Verification items for the finished model (mm, model axes). A direction names the side the tool comes from. Coordinates: 2 decimals unless noted, no trailing zeros. Order: outer loops, then holes, each group sorted by start corner. A loop starts at its lowest first (then second) coordinate and runs counter-clockwise, first axis right, second up. Notation, with made-up numbers: M 53,66 L 89,66 A14 ccw 89,70 Z; hole C 81,13 d7. An arc over 180 degrees is marked long. Return JSON: item names as keys, results as strings.
```python
from build123d import *

# Parameters (mm, degrees)
F1_DEPTH = 12
F0_W     = 17
F0_H     = 20
F2_DEPTH = 5
F3_R     = 4.99999
F4_R     = 2


# Not quite as in the source:
# - a fillet or chamfer is up to 0.001 mm smaller than in the source, because OpenCascade refuses the exact size


with BuildPart() as f1:
    # F0 (on Top) → F1 (new body)
    with BuildSketch(Plane.XY):
        Polygon((-43.5, 33), (43.5, 33), (43.5, 23), (46.5, 23), (46.5, 36), (-46.5, 36), (-46.5, -36), (46.5, -36), (46.5, -18), (43.5, -18), (43.5, -33), (-43.5, -33), align=None)
    extrude(amount=F1_DEPTH)

    # F0 (on Top) → F2 (join)
    with BuildSketch(Plane.XY):
        Polygon((43.5, 23), (43.5, 33), (-43.5, 33), (-43.5, -33), (43.5, -33), (43.5, -18), (23.5, -18), (23.5, 23), align=None)
        with Locations((-17, -18)):
            Rectangle(F0_W, F0_H, mode=Mode.SUBTRACT)
    extrude(amount=F2_DEPTH)

    # F3 (radius 5 in the source; OpenCascade refuses exactly that, so slightly less here)
    f3_edges = [f1.edges().sort_by_distance(p)[0] for p in [
        (23.5, 2.5, 0),
        (35, -18, 0),
        (35, 23, 0),
        (46.5, 29.5, 0),
        (46.5, -27, 0),
        (0, -36, 0),
        (0, 36, 0),
        (-46.5, 0, 0),
        (-46.5, 36, 6),
        (46.5, 36, 6),
        (46.5, -36, 6),
        (-46.5, -36, 6),
        (46.5, -18, 6),
        (46.5, 23, 6),
    ]]
    fillet(f3_edges, radius=F3_R)

    # F4
    f4_edges = [f1.edges().sort_by_distance(p)[0] for p in [
        (-25.5, -18, 5),
        (-17, -28, 5),
        (-17, -8, 5),
        (-8.5, -18, 5),
        (-17, -8, 0),
        (-25.5, -18, 0),
        (-17, -28, 0),
        (-8.5, -18, 0),
    ]]
    fillet(f4_edges, radius=F4_R)


solid = f1.part
```
Q1. Material ranges on line 1 along Y through (x, z) = (-4, 9); line 2 along X through (y, z) = (-24.5, 10.25); line 3 along Z through (x, y) = (-11.5, 28.5), recorded low to high.
Values:
{"line 1": "-36 to -33, 33 to 36", "line 2": "-46.5 to -43.5, 43.5 to 46.5", "line 3": "0 to 5"}
Q2. Cross-section at B-B, the plane y = -25. Record the boundary of the cut face in (x, z), and give its area (3 significant figures).
Values:
{"outline": "M -46.5,5 A5 ccw -41.5,0 L -27.5,0 A2 ccw -25.5,2 L -25.5,3 A2 ccw -27.5,5 L -43.5,5 L -43.5,12 L -46.5,12 Z; M -8.5,2 A2 ccw -6.5,0 L 41.5,0 A5 ccw 46.5,5 L 46.5,12 L 43.5,12 L 43.5,5 L -6.5,5 A2 ccw -8.5,3 Z", "area": "408 mm^2"}
Q3. Tool access check on faces 5 (the face through (-26.1, -17.83, 0.57)), 6 (the face through (-46.5, 0, 8)), 7 (the face through (-1, 0, 5)), 8 (the face through (45.07, -34.5, 8.55)), 9 (the face through (33, 24, 2)). Record the directions out of +Z, -Z, +X, -X, +Y, -Y that give a thin tool (end or side, any length) a straight path to the whole face; none if there is none.
Values:
{"face 5": "-Z", "face 6": "+Z, -Z, -X, +Y, -Y", "face 7": "+Z", "face 8": "+Z, -Z, +X, -Y", "face 9": "-Z, +X"}
Q4. Draft check along X on faces 1 (the face through (-1, -36, 8)), 2 (the face through (-45, -34.57, 8.55)), 3 (the face through (-16.85, -28.6, 4.43)), 4 (the face through (45, 29.52, 1.43)). Enter one of: pulls with the +X half, pulls with the -X half, needs draft (parallel to the pull), parting line crosses it, or undercut.
Values:
{"face 1": "needs draft", "face 2": "pulls with the -X half", "face 3": "undercut", "face 4": "pulls with the +X half"}
Q5. Cross-section at A-A, the plane x = -23.5. Record the boundary of the cut face in (y, z), and give its area (3 significant figures).
Values:
{"outline": "M -36,5 A5 ccw -31,0 L -30,0 A2 ccw -28,2 L -28,3 A2 ccw -30,5 L -33,5 L -33,12 L -36,12 Z; M -8,2 A2 ccw -6,0 L 31,0 A5 ccw 36,5 L 36,12 L 33,12 L 33,5 L -6,5 A2 ccw -8,3 Z", "area": "288 mm^2"}
Q6. Cross-section at C-C, the plane y = 29. Record the boundary of the cut face in (x, z), and give its area (3 significant figures).
Values:
{"outline": "M -46.5,5 A5 ccw -41.5,0 L 41.5,0 A5 ccw 46.5,5 L 46.5,12 L 43.5,12 L 43.5,5 L -43.5,5 L -43.5,12 L -46.5,12 Z", "area": "496 mm^2"}
Q7. Go/stop test with flat-tipped pins: pin 1 (3.5 mm diameter, centred on y = -10, z = 9, fed in from +X); pin 2 (1.1 mm diameter, centred on y = -19.5, z = 2.5, fed in from +X); pin 3 (4 mm diameter, centred on y = 13, z = 6, fed in from +X). Record where each tip stops, or that it passes through.
Values:
{"pin 1": "x = -43.5", "pin 2": "x = 44.81", "pin 3": "x = 23.5"}
Q8. Cross-section at D-D, the plane z = 8.75. Record the boundary of the cut face in (x, y), and give its area (3 significant figures).
Values:
{"outline": "M -46.5,-31 A5 ccw -41.5,-36 L 41.5,-36 A5 ccw 46.5,-31 L 46.5,-23 A5 ccw 43.5,-18.42 L 43.5,-33 L -43.5,-33 L -43.5,33 L 43.5,33 L 43.5,23.42 A5 ccw 46.5,28 L 46.5,31 A5 ccw 41.5,36 L -41.5,36 A5 ccw -46.5,31 Z", "area": "799 mm^2"}
